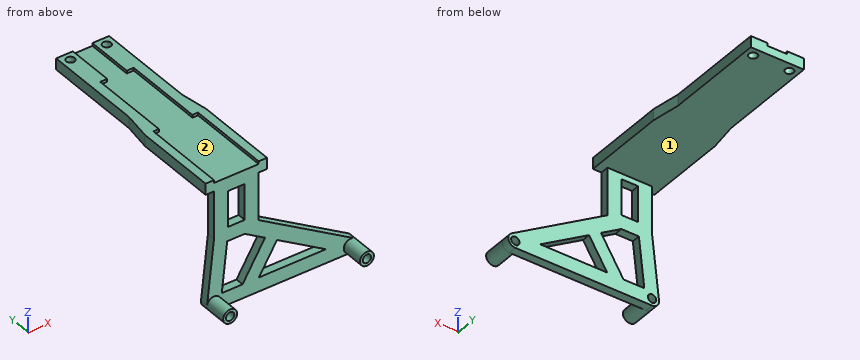
```python
from build123d import *
from OCP.BRepFilletAPI import BRepFilletAPI_MakeChamfer

# Parameters (mm, degrees)
ESQUISSE1_R             = 2.5
ESQUISSE1_R_2           = 1.5
BOSS_EXTRU_1_DEPTH      = 8
BOSS_EXTRU_1_2_DEPTH    = 8
ESQUISSE2_R             = 1.5
BOSS_EXTRU_2_DEPTH      = 3
ESQUISSE3_W             = 6
ESQUISSE3_H             = 12.810919071
ENL_V_MAT_EXTRU_1_DEPTH = 3
BOSS_EXTRU_3_START      = -3
BOSS_EXTRU_3_DEPTH      = 30
BOSS_EXTRU_5_DEPTH      = 29
BOSS_EXTRU_6_DEPTH      = 17
ESQUISSE7_R             = 1.5
ENL_V_MAT_EXTRU_2_DEPTH = 100.872418615
CHANFREIN1_SIZE         = 1.5
CHANFREIN1_SIZE_2       = 10


with BuildPart() as part:
    # Esquisse1 → Boss.-Extru.1 (new body)
    with BuildSketch(Plane(origin=(0, 0, 0), x_dir=(1, 0, 0), z_dir=(0, 1, 0))):
        with Locations(Location((-24.5, 0, 0), (0, 0, 270))):
            Circle(ESQUISSE1_R)
        with Locations(Location((-24.5, 0, 0), (0, 0, 270))):
            Circle(ESQUISSE1_R_2, mode=Mode.SUBTRACT)
    extrude(amount=BOSS_EXTRU_1_DEPTH)



with BuildPart() as body_2:
    # Esquisse1 → Boss.-Extru.1 2 (new body)
    with BuildSketch(Plane(origin=(0, 0, 0), x_dir=(1, 0, 0), z_dir=(0, 1, 0))):
        with Locations(Location((24.5, 0, 0), (0, 0, 270))):
            Circle(ESQUISSE1_R)
        with Locations(Location((24.5, 0, 0), (0, 0, 270))):
            Circle(ESQUISSE1_R_2, mode=Mode.SUBTRACT)
    extrude(amount=BOSS_EXTRU_1_2_DEPTH)


with BuildPart() as part_1:
    add(part.part)

    add(body_2.part)  # Boss.-Extru.2 merges body 2
    # Esquisse2 → Boss.-Extru.2 (add)
    with BuildSketch(Plane(origin=(0, 8, 0), x_dir=(1, 0, 0), z_dir=(0, 1, 0))):
        with BuildLine():
            Line((-24.5, 2.5), (24.5, 2.5))
            ThreePointArc((24.5, 2.5), (26.907248053, 0.674653105), (25.799245899, -2.13587455))
            Line((25.799245899, -2.13587455), (-8.5, -23))
            Line((-8.5, -23), (-8.5, -43))
            Line((-8.5, -43), (-24.5, -43))
            Line((-24.5, -43), (-24.5, -23))
            Line((-24.5, -23), (-26.985187688, -0.27173913))
            ThreePointArc((-26.985187688, -0.27173913), (-26.361363455, 1.668929623), (-24.5, 2.5))
        make_face()
        with Locations(Location((-24.5, 0, 0), (0, 0, 270))):
            Circle(ESQUISSE2_R, mode=Mode.SUBTRACT)
        with Locations(Location((24.5, 0, 0), (0, 0, 270))):
            Circle(ESQUISSE2_R, mode=Mode.SUBTRACT)
    extrude(amount=BOSS_EXTRU_2_DEPTH)

    # Esquisse3 → Enlèv. mat.-Extru.1 (cut)
    with BuildSketch(Plane(origin=(0, 11, 0), x_dir=(1, 0, 0), z_dir=(0, 1, 0))):
        Polygon((-6.206238259, -15.752308167), (-14.267576426, -2.5), (-21.711740643, -2.5), (-19.777554548, -20.189080929), (-13.5, -20.189080929), align=None)
        Polygon((-8.415172783, -2.5), (-1.934489158, -13.153816369), (15.579682155, -2.5), align=None)
        with Locations((-16.5, -31.594540464)):
            Rectangle(ESQUISSE3_W, ESQUISSE3_H)
    extrude(amount=-ENL_V_MAT_EXTRU_1_DEPTH, mode=Mode.SUBTRACT)

    # Esquisse4 → Boss.-Extru.3 (add)
    with BuildSketch(Plane(origin=(0, 11, 0), x_dir=(1, 0, 0), z_dir=(0, 1, 0)).offset(BOSS_EXTRU_3_START)):
        Polygon((-24.5, -44), (-27.5, -44), (-27.5, -40), (-24.5, -40), (-8.5, -40), (-5.5, -40), (-5.5, -44), (-8.5, -44), (-8.5, -43), (-24.5, -43), align=None)
    extrude(amount=BOSS_EXTRU_3_DEPTH)

    # Esquisse5 → Boss.-Extru.5 (add)
    with BuildSketch(Plane(origin=(0, 38, 0), x_dir=(1, 0, 0), z_dir=(0, 1, 0))):
        Polygon((-26, -44), (-22.5, -44), (-22.5, -43), (-10.5, -43), (-10.5, -44), (-7, -44), (-7, -40), (-26, -40), align=None)
    extrude(amount=BOSS_EXTRU_5_DEPTH)

    # Esquisse6 → Boss.-Extru.6 (add)
    with BuildSketch(Plane(origin=(0, 67, 0), x_dir=(1, 0, 0), z_dir=(0, 1, 0))):
        Polygon((-20, -44), (-20, -43), (-13, -43), (-13, -44), (-7, -44), (-7, -40), (-26, -40), (-26, -44), align=None)
    extrude(amount=BOSS_EXTRU_6_DEPTH)

    # Esquisse7 → Enlèv. mat.-Extru.2 (cut, through all)
    with BuildSketch(Plane.XY.offset(44)):
        with Locations((-23, 81)):
            Circle(ESQUISSE7_R)
        with Locations((-10, 81)):
            Circle(ESQUISSE7_R)
    extrude(amount=-ENL_V_MAT_EXTRU_2_DEPTH, mode=Mode.SUBTRACT)

    # Chanfrein1
    chanfrein1_edges_1 = [part_1.edges().sort_by_distance(p)[0] for p in [
        (-26, 38, 42),
    ]]
    chanfrein1_side_1 = [part_1.faces().sort_by_distance(p)[0] for p in [
        (-26.03, 38, 42),
    ]]
    chanfrein1_edges_2 = [part_1.edges().sort_by_distance(p)[0] for p in [
        (-7, 38, 42),
    ]]
    chanfrein1_side_2 = [part_1.faces().sort_by_distance(p)[0] for p in [
        (-6.97, 38, 42),
    ]]
    chanfrein1 = BRepFilletAPI_MakeChamfer(part_1.part.solid().wrapped)
    for e in chanfrein1_edges_1:
        chanfrein1.Add(CHANFREIN1_SIZE - 0.0001, CHANFREIN1_SIZE_2 - 0.0001, e.wrapped, chanfrein1_side_1[0].wrapped)
    for e in chanfrein1_edges_2:
        chanfrein1.Add(CHANFREIN1_SIZE - 0.0001, CHANFREIN1_SIZE_2 - 0.0001, e.wrapped, chanfrein1_side_2[0].wrapped)
    add(Compound.cast(chanfrein1.Shape()), mode=Mode.REPLACE)  # a hair under: the kernel refuses the full size


solid = part_1.part
```
Read the model definition and answer for the solid it produces. Units are mm, in the model's axes. Face numbers are marked on the shaded views. Give positions to 0.01 mm unless a question says otherwise; leave off trailing zeros. Write each loop counter-clockwise with the first axis right and the second up, starting at its lowest first coordinate (ties: lowest second). Pieces come first, ordered by that corner, then holes. Notation, with made-up numbers: (-18, 28.5) - (32, 28.5) arc R19 ccw to (32, 36.5) - close; hole circle Ø9 at (-27.5, 6). An arc over 180 degrees is marked (long way). Write item = value, one per line. Start each with the question number.
Item 1: Each of these flat-tipped pins is pushed along its axis until it touches: P1, Ø1.5, axis at x = -17.5, z = 20.5, coming from the -Y side; P2, Ø3.5, axis at y = 10, z = 27.5, coming from the +X side; P3, Ø2.5, axis at x = -10, y = 81, coming from the -Z side; P4, Ø4.5, axis at y = 57.5, z = 43, coming from the -X side. Where does it stop, or does it pass through?
Item 2: The mould has two halves that part along X. Classify the marked faces 1 and 2: +X half, -X half, draft (parallel to the pull), parting line (faces both ways), or undercut.
Item 3: Find the intervals of material crossed by probe 1 along X at (y, z) = (81, 41.6); probe 2 along X at (y, z) = (6.75, 0); probe 3 along Y at (x, z) = (-10, 42.05), in increasing order. Write a range as [from, to].
Item 4: Find section A-A (y = 81). Give the vertices of the cut face in (x, z), then the cut area to 3 significant figures.
Item 5: Find section B-B (z = 26.5). Give the vertices of the cut face in (x, y), then the cut area to 3 significant figures.
Item 6: Find section D-D (z = 6). Give the vertices of the cut face in (x, y).
Item 7: Find section C-C (y = 58). Give the vertices of the cut face in (x, z).
Response:
q1.P1 = 8
q1.P2 = -8.5
q1.P3 = through
q1.P4 = -26
q2.face_1 = draft
q2.face_2 = undercut
q3.probe_1 = [-26, -24.5], [-21.5, -11.5], [-8.5, -7]
q3.probe_2 = [-27, -26], [-23, -22], [22, 23], [26, 27]
q3.probe_3 = [8, 79.5], [82.5, 84]
q4.outline = (-26, 40) - (-24.5, 40) - (-24.5, 44) - (-26, 44) - close; (-21.5, 40) - (-11.5, 40) - (-11.5, 44) - (-13, 44) - (-13, 43) - (-20, 43) - (-20, 44) - (-21.5, 44) - close; (-8.5, 40) - (-7, 40) - (-7, 44) - (-8.5, 44) - close
q4.area = 45.0 mm²
q5.outline = (-24.5, 8) - (-19.5, 8) - (-19.5, 11) - (-24.5, 11) - close; (-13.5, 8) - (-8.5, 8) - (-8.5, 11) - (-13.5, 11) - close
q5.area = 30.0 mm²
q6.outline = (-26.36, 8) - (-21.33, 8) - (-21.33, 11) - (-26.36, 11) - close; (-12.14, 8) - (-6.29, 8) - (-6.29, 11) - (-12.14, 11) - close; (9.83, 8) - (19.45, 8) - (19.45, 11) - (9.83, 11) - close
q7.outline = (-26, 40) - (-7, 40) - (-7, 44) - (-10.5, 44) - (-10.5, 43) - (-22.5, 43) - (-22.5, 44) - (-26, 44) - close
